Geometry check sheet. Reference: the model listing, model coordinates, mm. A direction names the side the tool comes from. Round coordinates to 2 decimals unless told otherwise and drop trailing zeros. Write each loop counter-clockwise with the first axis right and the second up, starting at its lowest first coordinate (ties: lowest second). Pieces come first, ordered by that corner, then holes. Notation, with made-up numbers: (58, 15.5) - (110, 15.5) arc R14 ccw to (110, 32.5) - close; hole circle Ø7 at (8, 43.25). An arc over 180 degrees is marked (long way). Return JSON: item names as keys, results as strings.
```python
from build123d import *

# Parameters (mm, degrees)
SKETCH1_R                = 152.4
SKETCH1_R_2              = 127
BOSS_EXTRUDE1_DEPTH      = 38.1
SKETCH2_R                = 152.4
SKETCH2_R_2              = 139.7
CUT_EXTRUDE1_DEPTH       = 31.75
BOSS_EXTRUDE2_DEPTH      = 38.1
FILLET1_R                = 2.54
HOLE1_D                  = 8
HOLE1_DEPTH              = 87.532271537
CIRPATTERN1_COUNT        = 3
FILLET1_OF_CIRPATTERN1_R = 2.54


with BuildPart() as part:
    # Sketch1 → Boss-Extrude1 (new body)
    with BuildSketch(Plane(origin=(0, 0, 0), x_dir=(1, 0, 0), z_dir=(0, 1, 0))):
        Circle(SKETCH1_R)
        Circle(SKETCH1_R_2, mode=Mode.SUBTRACT)
    extrude(amount=BOSS_EXTRUDE1_DEPTH)

    # Sketch2 → Cut-Extrude1 (cut)
    with BuildSketch(Plane(origin=(0, 38.1, 0), x_dir=(1, 0, 0), z_dir=(0, 1, 0))):
        Circle(SKETCH2_R)
        Circle(SKETCH2_R_2, mode=Mode.SUBTRACT)
    extrude(amount=-CUT_EXTRUDE1_DEPTH, mode=Mode.SUBTRACT)

    # Sketch3 → Boss-Extrude2 (add, through all)
    with BuildSketch(Plane(origin=(0, 38.1, 0), x_dir=(1, 0, 0), z_dir=(0, 1, 0))):
        with BuildLine():
            Line((120.65, 25.4), (120.65, -25.4))
            Line((120.65, -25.4), (124.434078933, -25.4))
            ThreePointArc((124.434078933, -25.4), (127, 0), (124.434078933, 25.4))
            Line((124.434078933, 25.4), (120.65, 25.4))
        make_face()
    boss_extrude2 = extrude(amount=-BOSS_EXTRUDE2_DEPTH)

    # Fillet1
    fillet1_edges = [part.edges().sort_by_distance(p)[0] for p in [
        (124.434078933, 19.05, -25.4),
        (124.434078933, 19.05, 25.4),
    ]]
    fillet(fillet1_edges, radius=FILLET1_R)

    # Hole1
    with Locations(Plane(origin=(120.65, 0, -417.943859866), x_dir=(0, 0, 1), z_dir=(-1, 0, 0))):
        with Locations((400.481359866, 19.05), (435.406359866, 19.05)):
            hole1 = Hole(HOLE1_D / 2, depth=HOLE1_DEPTH)

    # CirPattern1: Boss-Extrude2, Hole1 ×3 about axis
    cirpattern1_axis = Axis((0, 0, 0), (0, 1, 0))
    for i in range(1, CIRPATTERN1_COUNT):
        add(boss_extrude2.rotate(cirpattern1_axis, i * 360 / CIRPATTERN1_COUNT))
        add(hole1.rotate(cirpattern1_axis, i * 360 / CIRPATTERN1_COUNT), mode=Mode.SUBTRACT)

    # Fillet1 of CirPattern1
    fillet1_of_cirpattern1_edges = [part.edges().sort_by_distance(p)[0] for p in [
        (-84.214084723, 19.05, -95.063073453),
        (-40.219994211, 19.05, -120.463073453),
        (-40.219994211, 19.05, 120.463073453),
        (-84.214084723, 19.05, 95.063073453),
    ]]
    fillet(fillet1_of_cirpattern1_edges, radius=FILLET1_OF_CIRPATTERN1_R)


solid = part.part
```
(1) Release check for a two-part mould opening along X. For faces 1 (the face through (-126.99, 18.78, -1.46)), 2 (the face through (67, 6.35, 123)), 3 (the face through (-110.86, 22.45, 85.01)) record: pulls with the +X half, pulls with the -X half, needs draft (parallel to the pull), parting line crosses it, or undercut.
Response values:
{"face 1": "undercut", "face 2": "needs draft", "face 3": "parting line crosses it"}
(2) Access from +Z, -Z, +X, -X, +Y, -Y to the whole of each face (thin tool, end or side, straight path). Record for faces 4 (the face through (129.982, 19.226, -13.466)), 5 (the face through (123, 0, -1)), 6 (the face through (-60.02, 19.32, 104.66)).
Response values:
{"face 4": "+X", "face 5": "+Z, -Z, +X, -X, -Y", "face 6": "+Y, -Y"}
(3) Gauge pin test, flat ends, axial feed: pin 1 (10 mm diameter, centred on x = 92, y = 22, fed in from -Z); pin 2 (0.7 mm diameter, centred on x = 121, y = 20.5, fed in from -Z); pin 3 (3 mm diameter, centred on y = 5.5, z = -48.5, fed in from +X). Record the tip position at first contact, or that the pin passes through.
Response values:
{"pin 1": "stops at z = -109.3", "pin 2": "stops at z = -70.42", "pin 3": "stops at x = 144.97"}
(4) Section check B-B, the plane y = 33.5. Enter the section's corners in (x, z).
Response values:
{"outline": "circle Ø279.4 at (0, 0); hole (-86.57, -92.92) arc R2.54 ccw to (-82.64, -92.33) - (-82.32, -91.79) - (-38.33, -117.19) - (-38.64, -117.73) arc R2.54 ccw to (-37.19, -121.43) arc R127 ccw to (123.76, -28.51) arc R2.54 ccw to (121.28, -25.4) - (120.65, -25.4) - (120.65, 25.4) - (121.28, 25.4) arc R2.54 ccw to (123.76, 28.51) arc R127 ccw to (-37.19, 121.43) arc R2.54 ccw to (-38.64, 117.73) - (-38.33, 117.19) - (-82.32, 91.79) - (-82.64, 92.33) arc R2.54 ccw to (-86.57, 92.92) arc R127 ccw to start"}
(5) Section check A-A, the plane z = 0. Enter the section's corners in (x, y).
Response values:
{"outline": "(-152.4, 0) - (-127, 0) - (-127, 38.1) - (-139.7, 38.1) - (-139.7, 6.35) - (-152.4, 6.35) - close; (120.65, 0) - (152.4, 0) - (152.4, 6.35) - (139.7, 6.35) - (139.7, 38.1) - (120.65, 38.1) - close"}
(6) Material ranges on line 1 along Z through (x, y) = (124.5, 19.05); line 2 along Z through (x, y) = (-1.5, 16); line 3 along Y through (x, z) = (-54.5, 137), recorded low to high. Write a range as [from, to].
Response values:
{"line 1": "z = [-63.37, -21.46], [-13.46, 13.46], [21.46, 63.37]", "line 2": "z = [-139.69, -126.99], [126.99, 139.69]", "line 3": "y = [0, 6.35]"}
(7) Section check C-C, the plane x = 0. Enter the section's corners in (y, z), plus the area to 3 significant figures.
Response values:
{"outline": "(0, -152.4) - (6.35, -152.4) - (6.35, -139.7) - (38.1, -139.7) - (38.1, -127) - (0, -127) - close; (0, 127) - (38.1, 127) - (38.1, 139.7) - (6.35, 139.7) - (6.35, 152.4) - (0, 152.4) - close", "area": "1,130 mm^2"}
